The model under review builds one solid part; all positions refer to its coordinate system, in mm. A direction names the side the tool comes from. Give positions to 0.01 mm unless a question says otherwise; leave off trailing zeros. Write each loop counter-clockwise with the first axis right and the second up, starting at its lowest first coordinate (ties: lowest second). Pieces come first, ordered by that corner, then holes. Notation, with made-up numbers: (1, 30.5) - (30, 30.5) arc R23 cw to (30, 67.5) - close; hole circle Ø2 at (41.25, 42). An arc over 180 degrees is marked (long way). Write item = value, one per line.
```python
from build123d import *

# Parameters (mm, degrees)
SKETCH1_R                    = 2.4
BOSS_EXTRUDE1_DEPTH          = 2
SKETCH2_W                    = 5
SKETCH2_H                    = 1
CUT_EXTRUDE1_DEPTH           = 51.038525021
EDGE_FLANGE1_STRIP_W         = 12
EDGE_FLANGE1_STRIP_H         = 2
EDGE_FLANGE1_STRIP_CUT_DEPTH = 15
EDGE_FLANGE1_DEPTH           = 15
EDGE_FLANGE2_STRIP_W         = 12
EDGE_FLANGE2_STRIP_H         = 2
EDGE_FLANGE2_STRIP_CUT_DEPTH = 6
EDGE_FLANGE2_DEPTH           = 6
EDGE_FLANGE3_STRIP_W         = 12
EDGE_FLANGE3_STRIP_H         = 2
EDGE_FLANGE3_STRIP_CUT_DEPTH = 6
EDGE_FLANGE3_DEPTH           = 6


# Sheet-metal steps are written as plain solids
with BuildPart() as part:
    # Sketch1 → Boss-Extrude1 (new body)
    with BuildSketch(Plane.XY):
        with BuildLine():
            Line((0.409525664, 7.488810902), (-19.507629857, 24.201288754))
            ThreePointArc((-19.507629857, 24.201288754), (-32.556888833, 27.318473412), (-27.221081173, 15.008755437))
            Line((-27.221081173, 15.008755437), (-18.272494906, 7.5))
            Line((-18.272494906, 7.5), (-40, 7.5))
            Line((-40, 7.5), (-40, -7.5))
            Line((-40, -7.5), (0, -7.5))
            ThreePointArc((0, -7.5), (7.497202204, -0.204839245), (0.409525664, 7.488810902))
        make_face()
        Circle(SKETCH1_R, mode=Mode.SUBTRACT)
        with Locations((-26.811555509, 22.497566339)):
            Circle(SKETCH1_R, mode=Mode.SUBTRACT)
    extrude(amount=BOSS_EXTRUDE1_DEPTH)

    # Sketch2 → Cut-Extrude1 (cut, through all)
    with BuildSketch(Plane.XY.offset(2)):
        with Locations((-23.5, 0)):
            Rectangle(SKETCH2_W, SKETCH2_H)
        with Locations((-8.5, 0)):
            Rectangle(SKETCH2_W, SKETCH2_H)
    extrude(amount=-CUT_EXTRUDE1_DEPTH, mode=Mode.SUBTRACT)

    # Edge-Flange1 strip (across the edge) → Edge-Flange1 strip cut (cut)
    with BuildSketch(Plane(origin=(-40, -7.5, 0), x_dir=(1, 0, 0), z_dir=(0, 1, 0))):
        with Locations((-2, -1)):
            Rectangle(EDGE_FLANGE1_STRIP_W, EDGE_FLANGE1_STRIP_H)
    extrude(amount=EDGE_FLANGE1_STRIP_CUT_DEPTH, mode=Mode.SUBTRACT)

    # Edge-Flange1 section (across the edge) → Edge-Flange1 (add)
    with BuildSketch(Plane(origin=(-40, -7.5, 0), x_dir=(1, 0, 0), z_dir=(0, 1, 0))):
        with BuildLine():
            Line((0, 2), (0, 8))
            Line((0, 8), (2, 8))
            Line((2, 8), (2, 2))
            ThreePointArc((2, 2), (2.585786438, 0.585786438), (4, 0))
            Line((4, 0), (4, -2))
            ThreePointArc((4, -2), (1.171572875, -0.828427125), (0, 2))
        make_face()
    extrude(amount=EDGE_FLANGE1_DEPTH)

    # Edge-Flange2 strip (across the edge) → Edge-Flange2 strip cut (cut)
    with BuildSketch(Plane(origin=(-40, 7.5, -2), x_dir=(0, -1, 0), z_dir=(0, 0, -1))):
        with Locations((-2, -1)):
            Rectangle(EDGE_FLANGE2_STRIP_W, EDGE_FLANGE2_STRIP_H)
    extrude(amount=EDGE_FLANGE2_STRIP_CUT_DEPTH, mode=Mode.SUBTRACT)

    # Edge-Flange2 section (across the edge) → Edge-Flange2 (add)
    with BuildSketch(Plane(origin=(-40, 7.5, -2), x_dir=(0, -1, 0), z_dir=(0, 0, -1))):
        with BuildLine():
            Line((0, 2), (0, 13))
            Line((0, 13), (2, 13))
            Line((2, 13), (2, 2))
            ThreePointArc((2, 2), (2.585786438, 0.585786438), (4, 0))
            Line((4, 0), (4, -2))
            ThreePointArc((4, -2), (1.171572875, -0.828427125), (0, 2))
        make_face()
    extrude(amount=EDGE_FLANGE2_DEPTH)

    # Edge-Flange3 strip (across the edge) → Edge-Flange3 strip cut (cut)
    with BuildSketch(Plane(origin=(-40, -7.5, -8), x_dir=(0, 1, 0), z_dir=(0, 0, 1))):
        with Locations((-2, -1)):
            Rectangle(EDGE_FLANGE3_STRIP_W, EDGE_FLANGE3_STRIP_H)
    extrude(amount=EDGE_FLANGE3_STRIP_CUT_DEPTH, mode=Mode.SUBTRACT)

    # Edge-Flange3 section (across the edge) → Edge-Flange3 (add)
    with BuildSketch(Plane(origin=(-40, -7.5, -8), x_dir=(0, 1, 0), z_dir=(0, 0, 1))):
        with BuildLine():
            Line((0, 2), (0, 12))
            Line((0, 12), (2, 12))
            Line((2, 12), (2, 2))
            ThreePointArc((2, 2), (2.585786438, 0.585786438), (4, 0))
            Line((4, 0), (4, -2))
            ThreePointArc((4, -2), (1.171572875, -0.828427125), (0, 2))
        make_face()
    extrude(amount=EDGE_FLANGE3_DEPTH)


solid = part.part
```
1. Insertion check: P1, Ø3, axis at x = -33.5, z = 0.5, coming from the +Y side; P2, Ø3, axis at x = -45, y = 5.5, coming from the +Z side; P3, Ø5, axis at x = -45.5, z = -5.5, coming from the +Y side. Each pin has a flat end and moves straight along its axis. Give the tip position at first contact, or say it passes through.
Findings below:
P1 = 27.91
P2 = -2
P3 = 7.5
2. Take a section at D-D on x = -35. Give the boundary of the cut face in (y, z).
Findings below:
outline = (-7.5, 0) - (7.5, 0) - (7.5, 2) - (-7.5, 2) - close
3. Take a section at B-B on y = 21. Give the boundary of the cut face in (x, z).
Findings below:
outline = (-34.16, 0) - (-28.69, 0) - (-28.69, 2) - (-34.16, 2) - close; (-24.94, 0) - (-15.69, 0) - (-15.69, 2) - (-24.94, 2) - close
4. Take a section at A-A on z = -5. Give the boundary of the cut face in (x, y).
Findings below:
outline = (-53, 5.5) - (-42, 5.5) arc R2 cw to (-40, 3.5) - (-40, -3.5) arc R2 cw to (-42, -5.5) - (-52, -5.5) - (-52, -7.5) - (-42, -7.5) arc R4 ccw to (-38, -3.5) - (-38, 3.5) arc R4 ccw to (-42, 7.5) - (-53, 7.5) - close
5. Machinability: for faces 4 (the flat face through (-38, 0, -5)), 5 (the flat face through (-29, 7.5, 1)), 6 (the flat face through (-47, 7.5, -5)), 7 (the flat face through (-24, -0.5, 1)), 8 (the cylindrical face through (-39.141, 6.297, -4.958)), which of the approach directions +Z, -Z, +X, -X, +Y, -Y give a long, thin tool a straight path to every point of the face, cutting with its end or side? Answer none if there is none.
Findings below:
face_4 = -Z, +X, +Y, -Y
face_5 = +Z, -Z, -X
face_6 = +Z, -Z, +X, -X, +Y
face_7 = +Z, -Z
face_8 = -Z, +X, +Y
6. Draft analysis for pull direction Z (two halves, no side actions). For faces 1 (the flat face through (-53, 7, -5)), 2 (the flat face through (-39, 0, -8)), 3 (the flat face through (-46, -6, -2)), state which applies: +Z half, -Z half, draft (parallel to the pull), parting line (faces both ways), or undercut.
Findings below:
face_1 = draft
face_2 = -Z half
face_3 = +Z half
7. For line 1 (Z direction, x = -23, y = 14); line 2 (X direction, y = 0.5, z = -6); line 3 (Y direction, x = 0, z = 0.8), list the stretches that pass through material, from the lowest coordinate up. Write a range as from..to.
Findings below:
line_1 = 0..2
line_2 = -40..-38
line_3 = -7.5..-2.4, 2.4..7.83
8. Take a section at C-C on x = -28. Give the boundary of the cut face in (y, z).
Findings below:
outline = (-7.5, 0) - (7.5, 0) - (7.5, 2) - (-7.5, 2) - close; (15.09, 0) - (20.41, 0) - (20.41, 2) - (15.09, 2) - close; (24.58, 0) - (29.9, 0) - (29.9, 2) - (24.58, 2) - close
